from build123d import *

# Parameters (mm, degrees)
ESQUISSE1_R                  = 2.75
BOSS_EXTRU_1_DEPTH           = 7.1
CONG_1_R                     = 3
CONG_2_R                     = 4
ENL_V_MAT_EXTRU_1_DEPTH      = 118.701866141
ENL_V_MAT_EXTRU_1_DEPTH_BACK = 78
CONG_3_R                     = 0.3


with BuildPart() as part:
    # Esquisse1 → Boss.-Extru.1 (new body)
    with BuildSketch(Plane.XY):
        Polygon((10, 95), (26.5, 105.4), (43, 95), (53, 95), (53, 0), (43, 0), (26.5, -10.4), (10, 0), (0, 0), (0, 95), align=None)
        with Locations((26.5, 100.71)):
            Circle(ESQUISSE1_R, mode=Mode.SUBTRACT)
        with Locations((26.5, -5.71)):
            Circle(ESQUISSE1_R, mode=Mode.SUBTRACT)
    extrude(amount=BOSS_EXTRU_1_DEPTH)

    # Congé1
    cong_1_edges = [part.edges().sort_by_distance(p)[0] for p in [
        (10, 95, 3.55),
        (26.5, 105.4, 3.55),
        (43, 95, 3.55),
        (43, 0, 3.55),
        (26.5, -10.4, 3.55),
        (10, 0, 3.55),
    ]]
    fillet(cong_1_edges, radius=CONG_1_R)

    # Congé2
    cong_2_edges = [part.edges().sort_by_distance(p)[0] for p in [
        (0, 95, 3.55),
        (53, 95, 3.55),
        (53, 0, 3.55),
        (0, 0, 3.55),
    ]]
    fillet(cong_2_edges, radius=CONG_2_R)

    # Esquisse3 → Enlèv. mat.-Extru.1 (cut, two sides: drawn at the far end of the back side and taken through both)
    with BuildSketch(Plane.XZ.offset(-ENL_V_MAT_EXTRU_1_DEPTH_BACK)):
        Polygon((5.154700538, 0), (4, 2), (4, 2.662509826), (10.145491142, 2.662509826), (10.145491142, 2.062509826), (8.954700538, 0), align=None)
        Polygon((44.009209397, 0), (42.854508858, 2), (42.854508858, 2.662509826), (49, 2.662509826), (49, 2.062509826), (47.809209397, 0), align=None)
    extrude(amount=ENL_V_MAT_EXTRU_1_DEPTH + ENL_V_MAT_EXTRU_1_DEPTH_BACK, mode=Mode.SUBTRACT)

    # Congé3
    cong_3_edges = [part.edges().sort_by_distance(p)[0] for p in [
        (44.009209397, 39, 0),
        (47.809209397, 39, 0),
        (8.954700538, 39, 0),
        (5.154700538, 39, 0),
    ]]
    fillet(cong_3_edges, radius=CONG_3_R)


solid = part.part
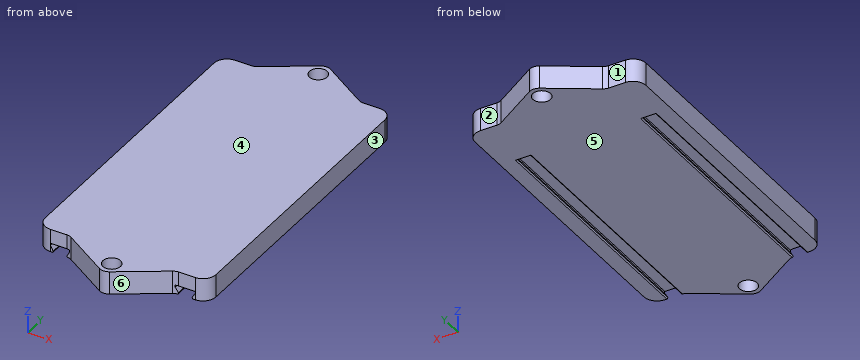
The model under review builds one solid part; all positions refer to its coordinate system, in mm. Face numbers are marked on the shaded views. A direction names the side the tool comes from. Coordinates: 2 decimals unless noted, no trailing zeros. Loops run counter-clockwise (first coordinate to the right, second up) from the corner with the lowest first, then second, coordinate; pieces in that order, holes last.
(1) Wall thickness on L1, parallel to X at y = 28.5, z = 0.5; L2, parallel to Y at x = 46, z = 1.75; L3, parallel to Y at x = 4, z = 1.5: over which ranges is each line inside the solid? List them lowest first.
Determined:
L1: x = 0 to 4.87, 9.24 to 43.72, 48.1 to 53
L2: y = 78 to 95
L3: y = 0 to 95
(2) Consider section A-A, the plane z = 5.75. Give the boundary of the cut face in (x, y).
Determined:
outline: (0, 4) arc R4 ccw to (4, 0) - (9.13, 0) arc R3 cw to (10.73, -0.46) - (24.9, -9.39) arc R3 ccw to (28.1, -9.39) - (42.27, -0.46) arc R3 cw to (43.87, 0) - (49, 0) arc R4 ccw to (53, 4) - (53, 91) arc R4 ccw to (49, 95) - (43.87, 95) arc R3 cw to (42.27, 95.46) - (28.1, 104.39) arc R3 ccw to (24.9, 104.39) - (10.73, 95.46) arc R3 cw to (9.13, 95) - (4, 95) arc R4 ccw to (0, 91) - close; hole circle Ø5.5 at (26.5, -5.71); hole circle Ø5.5 at (26.5, 100.71)
(3) Consider section C-C, the plane y = 100.71. Give the boundary of the cut face in (x, z), plus the area to 3 significant figures.
Determined:
outline: (19.06, 0) - (23.75, 0) - (23.75, 7.1) - (19.06, 7.1) - close; (29.25, 0) - (33.94, 0) - (33.94, 7.1) - (29.25, 7.1) - close
area: 66.6 mm2
(4) Consider section B-B, the plane x = 26.5. Give the boundary of the cut face in (y, z).
Determined:
outline: (-9.85, 0) - (-8.46, 0) - (-8.46, 7.1) - (-9.85, 7.1) - close; (-2.96, 0) - (97.96, 0) - (97.96, 7.1) - (-2.96, 7.1) - close; (103.46, 0) - (104.85, 0) - (104.85, 7.1) - (103.46, 7.1) - close
(5) Insertion check: P1, Ø3, axis at x = 6, z = 1.5, coming from the -Y side; P2, Ø4, axis at x = 45.5, z = 4.5, coming from the +Y side; P3, Ø1.3, axis at x = 46.5, z = 1, coming from the -Y side. Each pin has a flat end and moves straight along its axis. Give the tip position at first contact, or say it passes through.
Determined:
P1: stops at y = 0
P2: stops at y = 95.02
P3: stops at y = 78
(6) Draft analysis for pull direction Z (two halves, no side actions). For the marked faces 4, 5 and 6, state which applies: +Z half, -Z half, draft (parallel to the pull), parting line (faces both ways), or undercut.
Determined:
face 4: +Z half
face 5: -Z half
face 6: draft
(7) Consider section D-D, the plane y = 28. Give the boundary of the cut face in (x, z), plus the area to 3 significant figures.
Determined:
outline: (0, 0) - (4.64, 0) arc R0.3 ccw to (4.89, 0.45) - (4, 2) - (4, 2.66) - (10.15, 2.66) - (10.15, 2.06) - (9.21, 0.45) arc R0.3 ccw to (9.47, 0) - (43.49, 0) arc R0.3 ccw to (43.75, 0.45) - (42.85, 2) - (42.85, 2.66) - (49, 2.66) - (49, 2.06) - (48.07, 0.45) arc R0.3 ccw to (48.33, 0) - (53, 0) - (53, 7.1) - (0, 7.1) - close
area: 348 mm2
(8) Tool access review of the marked faces 1, 2 and 3: name each direction out of +Z, -Z, +X, -X, +Y, -Y from which nothing blocks a thin tool from reaching the whole face with its end or side.
Determined:
face 1: +Z, -Z, -X, +Y
face 2: +Z, -Z, +X, +Y
face 3: +Z, -Z, +X, +Y, -Y
